Verification items for this drawing (mm, ordinates from the low corner). A direction names the side the tool comes from. Coordinates: 2 decimals unless noted, no trailing zeros. Loops run counter-clockwise (first coordinate to the right, second up) from the corner with the lowest first, then second, coordinate; pieces in that order, holes last. Notation, with made-up numbers: M 9,-37 L 28,-37 A21 cw 28,-26 Z; hole C -35.5,34.25 d9. An arc over 180 degrees is marked long. Write each question's results on one line, items separated by ' | '. Start each with the question number.
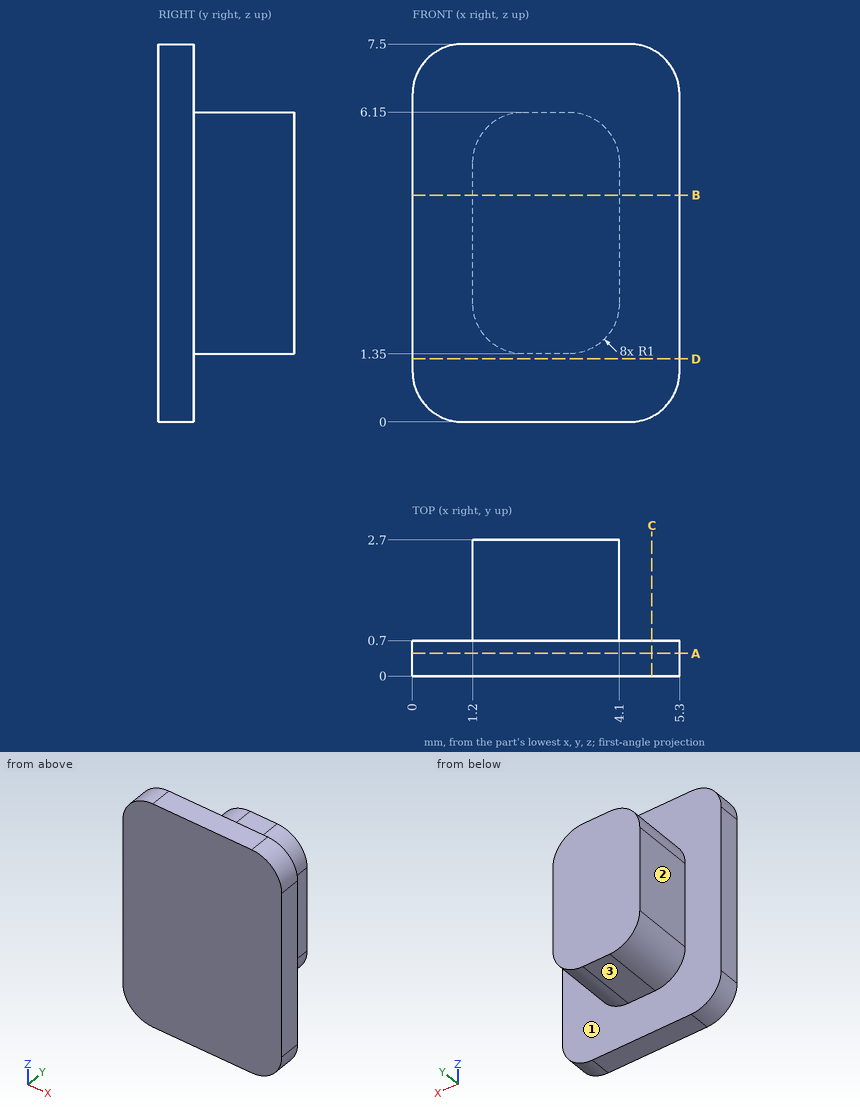
Item 1: Depth check by flat-ended pin: P1, Ø0.7, axis at x = 2.5, y = 1.5, coming from the +Z side; P2, Ø1, axis at x = 2.5, y = 2, coming from the -Z side; P3, Ø0.6, axis at y = 1.5, z = 4.5, coming from the +X side. Enter the tip coordinate at first touch or a pass-through.
Item 2: Thickness scan on line 1 (X direction, y = 1.7, z = 4.25); line 2 (Y direction, x = 0.5, z = 2.25); line 3 (Z direction, x = 2.1, y = 2.5). Record the ranges inside material, lowest first.
Item 3: Section check D-D (z = 1.25). Record the cut outline in (x, y), plus the area to 3 significant figures.
Item 4: Tool access check on the marked faces 1, 2 and 3. Record the directions out of +Z, -Z, +X, -X, +Y, -Y that give a thin tool (end or side, any length) a straight path to the whole face; none if there is none.
Item 5: Section check B-B (z = 4.5). Record the cut outline in (x, y).
Item 6: Section check C-C (x = 4.75). Record the cut outline in (y, z), plus the area to 3 significant figures.
Item 7: Section check A-A (y = 0.45). Record the cut outline in (x, z).
Computed values:
1) P1: stops at z = 6.15 | P2: stops at z = 1.35 | P3: stops at x = 4.1
2) line 1: x = 1.2 to 4.1 | line 2: y = 0 to 0.7 | line 3: z = 1.36 to 6.14
3) outline: M 0,0 L 5.3,0 L 5.3,0.7 L 0,0.7 Z | area: 3.71 mm²
4) face 1: +Y | face 2: +Z, -Z, -X, +Y | face 3: -Z, +X, -X, +Y
5) outline: M 0,0 L 5.3,0 L 5.3,0.7 L 4.1,0.7 L 4.1,2.7 L 1.2,2.7 L 1.2,0.7 L 0,0.7 Z
6) outline: M 0,0.11 L 0.7,0.11 L 0.7,7.39 L 0,7.39 Z | area: 5.10 mm²
7) outline: M 0,1 A1 ccw 1,0 L 4.3,0 A1 ccw 5.3,1 L 5.3,6.5 A1 ccw 4.3,7.5 L 1,7.5 A1 ccw 0,6.5 Z
